The drawing under review shows one solid part. Ordinate dimensions are in mm from its lowest x, y, z. Coordinates: 2 decimals unless noted, no trailing zeros.
Q1. To check wall thickness, follow probe 1 along X at (y, z) = (4.5, 60); probe 2 along X at (y, z) = (1, 53.5) (1 decimal); probe 3 along Z at (x, y) = (50.8, 3.75) (1 decimal). State the ranges of each line that lie inside material, in increasing order.
Q2. Add section C-C, the plane x = 12.7. Give the number of separate pieces and of enclosed holes in the cut face.
Q3. Clearance check with a flat-ended pin moving along its axis: pin 1 Ø3 at (x, z) = (11.95, 3.2) entering from -Y. State where the tip first meets the part, or that it passes through.
Q4. The part is to be moulded in two halves that separate along Z. For the marked faces 1, 2 and 3, say which applies: +Z half, -Z half, draft (parallel to the pull), parting line (faces both ways), or undercut.
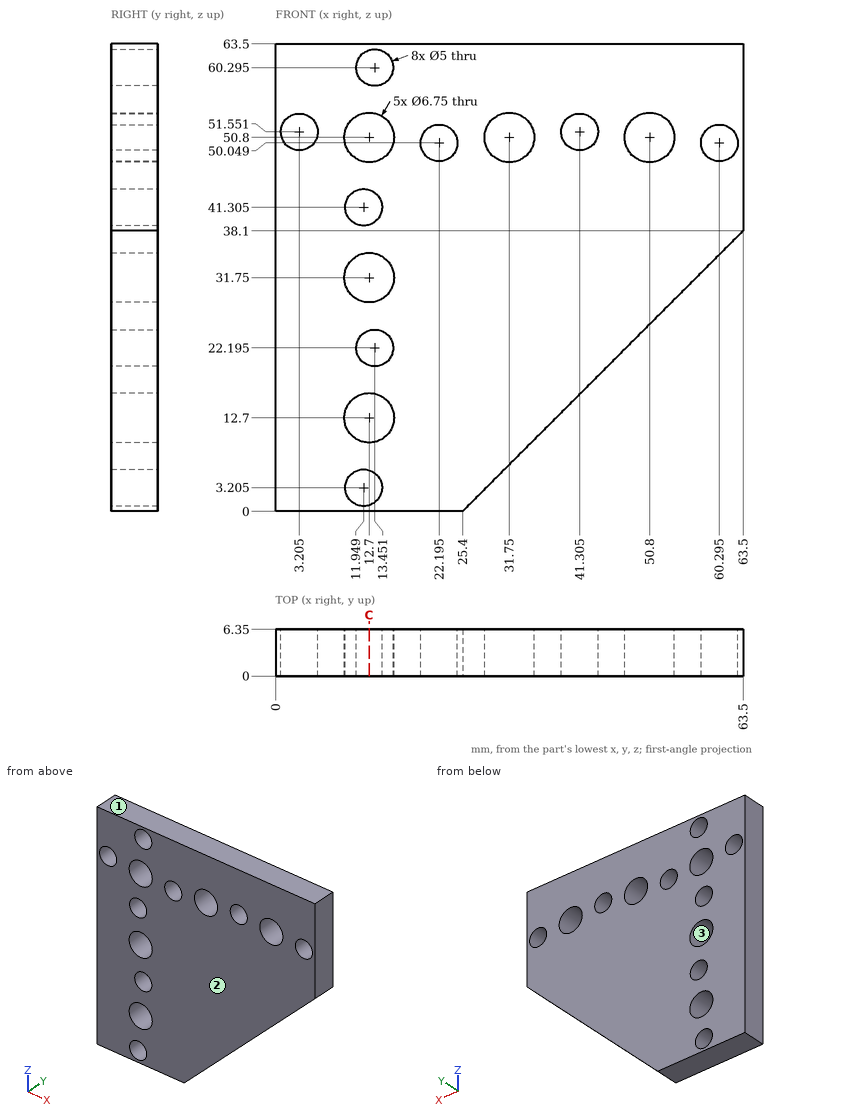
Here are the results:
1. probe 1: x = 0 to 10.97, 15.93 to 63.5
1. probe 2: x = 0 to 1.6, 4.8 to 10.7, 14.7 to 29.7, 33.8 to 39.7, 42.9 to 48.8, 52.8 to 63.5
1. probe 3: z = 25.4 to 47.4, 54.2 to 63.5
2. separate pieces: 8
2. enclosed holes: 0
3. pin 1: passes through
4. face 1: +Z half
4. face 2: draft
4. face 3: undercut
